Autodesk Inventor part; units mm, degrees
ref_plane "YZ Plane" through (0, 0, 0) normal (1, 0, 0) x (0, 1, 0)
ref_plane "XZ Plane" through (0, 0, 0) normal (0, 1, 0) x (-1, 0, 0)
ref_plane "XY Plane" through (0, 0, 0) normal (0, 0, 1) x (1, 0, 0)
sketch "Sketch1" plane through (0, 0, 0) normal (0, 1, 0) x (-1, 0, 0)
  line L0 (13.4736, 15.4721) -> (-11.9264, 15.4721)
  line L1 (-11.9264, 15.4721) -> (-11.9264, -9.9279)
  line L2 (-11.9264, -9.9279) -> (13.4736, -9.9279)
  line L3 (13.4736, -9.9279) -> (13.4736, 15.4721)
  point P0 (0, 0)
  dimension "d0" = 25.4
  dimension "d1" = 25.4
extrude "Extrusion1" add sketch "Sketch1" along normal blind 609.6
shell "Shell1" thickness 3.175 removed faces 1 at (3.4597, 609.6, 7.0054)
sketch "Sketch2" plane through (0, 609.6, 0) normal (0, 1, 0) x (1, 0, 0)
  line L0 (-10.2986, -12.2971) -> (8.7514, -12.2971)
  line L1 (8.7514, -12.2971) -> (8.7514, 6.7529)
  line L2 (8.7514, 6.7529) -> (-10.2986, 6.7529)
  line L3 (-10.2986, 6.7529) -> (-10.2986, -12.2971)
  point P0 (0, 0)
extrude "Extrusion2" cut sketch "Sketch2" against normal blind 609.6
sketch "Sketch3" plane through (-13.4736, 0, 15.4721) normal (0, 0, 1) x (1, 0, 0)
  line L0 (38.1, 608.6348) -> (0, 608.6348)
  circle A0 centre (12.7, 12.7) radius 3.3655
  circle A1 centre (12.7, 342.9) radius 3.3655
  circle A2 centre (12.7, 595.9348) radius 3.3655
  line L1 (0, 557.8348) -> (0, 608.6348)
  line L2 (0, 50.8) -> (0, 0)
  line L3 (12.7, 342.9) -> (0, 304.3174) construction
  line L4 (0, 317.5) -> (0, 368.3)
  line L5 (0, 129.921) -> (12.7, 129.921) construction
  circle A3 centre (12.7, 129.921) radius 3.3655
  circle A4 centre (12.7, 174.371) radius 3.3655
  line L6 (9.3413, 197.482) -> (9.3413, 204.213)
  line L7 (16.0611, 204.488) -> (16.0611, 197.3435)
  arc A5 (16.0611, 204.488) -> (9.3413, 204.213) centre (12.6956, 204.488) ccw
  arc A6 (9.3413, 197.482) -> (16.0611, 197.3435) centre (12.6974, 197.231) ccw
  circle A7 centre (12.7, 217.188) radius 3.3655
  line L8 (0, 0) -> (0, 609.6)
  point P0 (13.4736, 0)
  dimension "d7" = 38.1
  dimension "d20" = 12.7
  dimension "d29" = 12.7
  dimension "d30" = 6.731
  dimension "d31" = 3.3655
  dimension "d32" = 3.3655
  dimension "d33" = 6.731
  dimension "d34" = 12.7
  dimension "d36" = 90
  dimension "d37" = 90
  dimension "d40" = 478.7138
  dimension "d44" = 404.1468
  dimension "d45" = 411.2913
  dimension "d48" = 434.2638
  dimension "d49" = 50.8
  dimension "d50" = 240.3348
  dimension "d51" = 291.1348
  dimension "d52" = 557.8348
extrude "Extrusion3" cut sketch "Sketch3" against normal blind 76.2
sketch "Sketch4" plane through (-13.4736, 0, 15.4721) normal (0, 0, 1) x (1, 0, 0)
  line L0 (0, 0) -> (25.4, 0)
  line L1 (25.4, 0) -> (25.4, 25.4)
  line L2 (25.4, 25.4) -> (0, 25.4)
  line L3 (0, 25.4) -> (0, 0)
  point P0 (13.4736, 0)
  dimension "d55" = 25.4
  dimension "d56" = 25.4
extrude "Extrusion4" cut sketch "Sketch4" against normal blind 25.4
properties part number "ClawArmBeam"
Here's how the part is built. I have some questions about the finished solid (model axes, mm). A direction names the side the tool comes from. Round coordinates to 2 decimals unless told otherwise and drop trailing zeros. Write each loop counter-clockwise with the first axis right and the second up, starting at its lowest first coordinate (ties: lowest second). Pieces come first, ordered by that corner, then holes.
Q1. Which directions (+Z, -Z, +X, -X, +Y, -Y) give clear straight access to the entire face, cutting with the end or side of a thin tool? Please do faces 1 (the flat face through (-1, 322, -6.753)), 2 (the flat face through (11, 609.6, 3)).
Q2. If we section it at B-B on y = 364: Write out the boundary of the cut face in (x, z).
Q3. Please list where these lines run through material, in increasing order: probe 1 along Z at (x, y) = (-4, 153); probe 2 along X at (y, z) = (105, 8.5).
Q4. If we mould it in two halves opening along Z, with no side actions, what happens to faces 3 (the flat face through (8.751, 322, 3)), 4 (the flat face through (11.926, 313, 3)), 5 (the flat face through (-1, 313, -9.928))? For each: +Z half, -Z half, draft (parallel to the pull), parting line (faces both ways), or undercut.
Q5. If we section it at A-A on z = 3.75: Write out the boundary of the cut face in (x, y), plus the area to 3 significant figures.
Q6. Will this pin go through, and if not, where does the flat tip stop? P1, Ø5.5, axis at x = -0.77, y = 595.93, coming from the +Z side.
Answer below:
1. face 1: +Y, -Y
1. face 2: +Z, -Z, +X, -X, +Y
2. outline: (-13.47, -9.93) - (11.93, -9.93) - (11.93, 15.47) - (-13.47, 15.47) - close; hole (-10.3, -6.75) - (8.75, -6.75) - (8.75, 12.3) - (-10.3, 12.3) - close
3. probe 1: z = -9.93 to -6.75, 12.3 to 15.47
3. probe 2: x = -13.47 to -10.3, 8.75 to 11.93
4. face 3: undercut
4. face 4: draft
4. face 5: -Z half
5. outline: (-13.47, 25.4) - (-10.3, 25.4) - (-10.3, 609.6) - (-13.47, 609.6) - close; (8.75, 25.4) - (11.93, 25.4) - (11.93, 609.6) - (8.75, 609.6) - close
5. area: 3,710 mm2
6. P1: passes through
